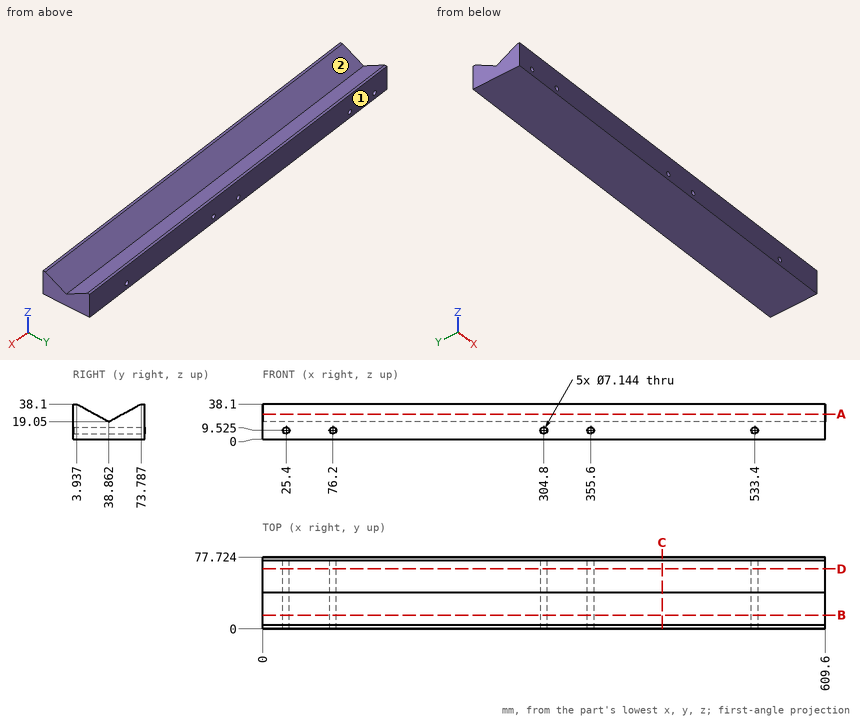
Could you check a few things on this drawing? It's one solid part, dimensions in mm from its lowest x, y, z. A direction names the side the tool comes from. Round coordinates to 2 decimals unless told otherwise and drop trailing zeros. Order: outer loops, then holes, each group sorted by start corner. A loop starts at its lowest first (then second) coordinate and runs counter-clockwise, first axis right, second up. Notation, with made-up numbers: M -30.75,-37.5 L -7.75,-37.5 A29 ccw -7.75,-5.5 Z; hole C 42,43 d11. An arc over 180 degrees is marked long. Return JSON: item names as keys, results as strings. Group by question number.
1. On a 3-axis mill with a long thin cutter (end or side, diameter ignored), from which of +Z, -Z, +X, -X, +Y, -Y can I reach the whole of each face in a straight line? I mean the marked faces 1 and 2. Say none if no direction works.
2. If we section it at A-A on z = 27: List the corners of the cut face in (x, y) for me.
3. If we section it at D-D on y = 65: List the corners of the cut face in (x, z) for me (1 decimal), then the cut area to 3 significant figures.
4. Please list where these lines run through material, in increasing order: probe 1 along X at (y, z) = (8, 9.5); probe 2 along X at (y, z) = (21.5, 7) (1 decimal); probe 3 along Z at (x, y) = (304.8, 31).
5. If we section it at B-B on y = 15: List the corners of the cut face in (x, z) for me (1 decimal), then the cut area to 3 significant figures.
6. If we section it at C-C on x = 433: List the corners of the cut face in (y, z) for me, then the cut area to 3 significant figures.
7. I'm going to push flat-ended pins straight in: pin 1 Ø5.5 at (x, z) = (355.6, 9.525) entering from +Y; pin 2 Ø6 at (x, y) = (250, 16.5) entering from -Z; pin 3 Ø2 at (x, y) = (144.5, 54.5) entering from +Z (1 decimal); pin 4 Ø6 at (x, y) = (504.5, 31) entering from +Z (1 decimal). Where does each tip first touch, or does it pass through?
Reply:
{
 "1": {"face 1": "+Z, -Z, +X, -X, +Y", "face 2": "+Z, +X, -X"},
 "2": {"outline": "M 0,0 L 609.6,0 L 609.6,24.29 L 0,24.29 Z; M 0,53.44 L 609.6,53.44 L 609.6,77.72 L 0,77.72 Z"},
 "3": {"outline": "M 0,0 L 609.6,0 L 609.6,33.3 L 0,33.3 Z; hole C 25.4,9.5 d7.1; hole C 76.2,9.5 d7.1; hole C 304.8,9.5 d7.1; hole C 355.6,9.5 d7.1; hole C 533.4,9.5 d7.1", "area": "20,100 mm^2"},
 "4": {"probe 1": "0 to 21.83, 28.97 to 72.63, 79.77 to 301.23, 308.37 to 352.03, 359.17 to 529.83, 536.97 to 609.6", "probe 2": "0 to 22.9, 27.9 to 73.7, 78.7 to 302.3, 307.3 to 353.1, 358.1 to 530.9, 535.9 to 609.6", "probe 3": "0 to 5.95, 13.1 to 23.34"},
 "5": {"outline": "M 0,0 L 609.6,0 L 609.6,32.1 L 0,32.1 Z; hole C 25.4,9.5 d7.1; hole C 76.2,9.5 d7.1; hole C 304.8,9.5 d7.1; hole C 355.6,9.5 d7.1; hole C 533.4,9.5 d7.1", "area": "19,300 mm^2"},
 "6": {"outline": "M 0,0 L 77.72,0 L 77.72,38.1 L 73.79,38.1 L 38.86,19.05 L 3.94,38.1 L 0,38.1 Z", "area": "2,300 mm^2"},
 "7": {"pin 1": "through", "pin 2": "z = 0", "pin 3": "z = 28.1", "pin 4": "z = 25"}
}
